```python
from build123d import *

# Parameters (mm, degrees)
SKETCH011_W     = 52
SKETCH011_H     = 30
SKETCH011_W_2   = 46
SKETCH011_H_2   = 24
PAD011_DEPTH    = 8
SKETCH012_R     = 1.5
POCKET_DEPTH    = 52.001
SKETCH013_R     = 1.5
POCKET001_DEPTH = 30.001


with BuildPart() as part:
    # Sketch011 → Pad011 (new body)
    with BuildSketch(Plane.YZ):
        with Locations((26, 15)):
            Rectangle(SKETCH011_W, SKETCH011_H)
        with Locations((26, 15)):
            Rectangle(SKETCH011_W_2, SKETCH011_H_2, mode=Mode.SUBTRACT)
    extrude(amount=PAD011_DEPTH)

    # Sketch012 (on Face2 of Pad011) → Pocket (cut, through all)
    with BuildSketch(Plane.ZX.offset(52)):
        with Locations((6, 4)):
            Circle(SKETCH012_R)
        with Locations((24, 4)):
            Circle(SKETCH012_R)
    extrude(amount=-POCKET_DEPTH, mode=Mode.SUBTRACT)

    # Sketch013 (on Face1 of Pocket) → Pocket001 (cut, through all)
    with BuildSketch(Plane.YX):
        with Locations((10, 4)):
            Circle(SKETCH013_R)
        with Locations((42, 4)):
            Circle(SKETCH013_R)
    extrude(amount=-POCKET001_DEPTH, mode=Mode.SUBTRACT)


solid = part.part
```
CAD build for the part. Positions are in the model's coordinates, mm. A direction names the side the tool comes from. Coordinates: 2 decimals unless noted, no trailing zeros. Order: outer loops, then holes, each group sorted by start corner. A loop starts at its lowest first (then second) coordinate and runs counter-clockwise, first axis right, second up. Notation, with made-up numbers: (15.5, 78.25) -> (27.5, 78.25) arc R8 cw to (27.5, 89.25) -> close; hole circle Ø4 at (-34.75, 31). An arc over 180 degrees is marked (long way). Use one line per item in the form item = value. Start each with the question number.
1) Drill centre lines: L1, parallel to Z at x = 6.5, y = 31; L2, parallel to X at y = 50.9, z = 6; L3, parallel to Y at x = 0.75, z = 21.5. Where is each one in solid material? Low to high. Write a range as [from, to].
2) Band-saw the part on A-A on z = 8.25. Give the cut face in (x, y), then the cut area to 3 significant figures.
3) Band-saw the part on C-C on z = 24. Give the cut face in (x, y), then the cut area to 3 significant figures.
4) Pull direction X, two halves, no side cores. Call faces 1 (the flat face through (8, 22, 2.8)), 2 (the flat face through (4, 0, 15)), 3 (the cylindrical face through (4.07, 40.5, 1.48)): +X half, -X half, draft (parallel to the pull), parting line (faces both ways), or undercut.
5) Tool access for faces 4 (the flat face through (4, 26, 27)), 5 (the flat face through (4, 52, 15)): list every direction of +Z, -Z, +X, -X, +Y, -Y with a clear straight run to the whole face (end or side of a thin tool).
6) Band-saw the part on D-D on x = 2. Give the cut face in (y, z), then the cut area to 3 significant figures.
7) Drop flat-ended pins along their axis: pin 1 (3.5 mm diameter, centred on x = 4, y = 10, fed in from +Z); pin 2 (2.5 mm diameter, centred on x = 4, y = 42, fed in from +Z). Give the stop position or say it passes through.
8) Band-saw the part on B-B on y = 29. Give the cut face in (x, z), then the cut area to 3 significant figures.
Entries:
q1.L1 = [0, 3], [27, 30]
q1.L2 = [0, 2.5], [5.5, 8]
q1.L3 = [0, 3], [49, 52]
q2.outline = (0, 0) -> (8, 0) -> (8, 3) -> (0, 3) -> close; (0, 49) -> (8, 49) -> (8, 52) -> (0, 52) -> close
q2.area = 48.0 mm2
q3.outline = (0, 0) -> (2.5, 0) -> (2.5, 3) -> (0, 3) -> close; (0, 49) -> (2.5, 49) -> (2.5, 52) -> (0, 52) -> close; (5.5, 0) -> (8, 0) -> (8, 3) -> (5.5, 3) -> close; (5.5, 49) -> (8, 49) -> (8, 52) -> (5.5, 52) -> close
q3.area = 30.0 mm2
q4.face_1 = +X half
q4.face_2 = draft
q4.face_3 = undercut
q5.face_4 = +X, -X
q5.face_5 = +Z, -Z, +X, -X, +Y
q6.outline = (0, 0) -> (52, 0) -> (52, 30) -> (0, 30) -> close; hole (3, 3) -> (49, 3) -> (49, 27) -> (3, 27) -> close
q6.area = 456 mm2
q7.pin_1 = 30
q7.pin_2 = through
q8.outline = (0, 0) -> (8, 0) -> (8, 3) -> (0, 3) -> close; (0, 27) -> (8, 27) -> (8, 30) -> (0, 30) -> close
q8.area = 48.0 mm2
